Here's how the part is built. I have some questions about the finished solid (model axes, mm). A direction names the side the tool comes from. Round coordinates to 2 decimals unless told otherwise and drop trailing zeros. Write each loop counter-clockwise with the first axis right and the second up, starting at its lowest first coordinate (ties: lowest second). Pieces come first, ordered by that corner, then holes. Notation, with made-up numbers: M 79,-23 L 109,-23 A24 ccw 109,7 Z; hole C 0.5,79.25 d6. An arc over 180 degrees is marked long. Use one line per item in the form item = value. Start each with the question number.
Q1. I'm going to push flat-ended pins straight in: pin 1 Ø1 at (x, z) = (-1.5, 0) entering from -Y; pin 2 Ø1.1 at (x, y) = (-1.5, 7) entering from -Z; pin 3 Ø2 at (x, z) = (2, -0.5) entering from +Y; pin 4 Ø0.7 at (y, z) = (6.5, 1) entering from +X. Where does each tip first touch, or does it pass through?
Q2. I want a section at B-B on z = 0. List the corners of the cut face in (x, y) for me, and give its area (3 significant figures).
Q3. I need wall thicknesses on line 1 along Z through (x, y) = (-0.8, 6.25); line 2 along X through (y, z) = (6.25, -1.1); line 3 along X through (y, z) = (6.5, -1.2). Which ranges of each line are inside material? Lowest first, please. Write a range as from..to.
Q4. I want a section at D-D on z = -0.75. List the corners of the cut face in (x, y) for me.
Q5. We'd pull the mould along X, two halves only. Please class faces 5 (the face through (1, 7, -0.5)), 6 (the face through (0.5, 7, -1)), 7 (the face through (-1.5, 2.46, -0.07)): +X half, -X half, draft (parallel to the pull), parting line (faces both ways), or undercut.
Q6. For faces 1 (the face through (0, 0, 0)), 2 (the face through (0.5, 7, 1)), 3 (the face through (1, 7, 0.5)), 4 (the face through (2, 5, 0)), which set-ups out of +Z, -Z, +X, -X, +Y, -Y let a thin tool reach every point of the face, with its end or its side?
Q7. I want a section at A-A on x = 0. List the corners of the cut face in (y, z) for me.
Q8. I want a section at C-C on y = 2.75. List the corners of the cut face in (x, z) for me.
```python
from build123d import *

# Parameters (mm, degrees)
SKETCH1_R           = 1.5
BOSS_EXTRUDE1_DEPTH = 5
REVOLVE1_ANGLE      = 180
CUT_EXTRUDE1_DEPTH  = 2


with BuildPart() as part:
    # Sketch1 → Boss-Extrude1 (new body)
    with BuildSketch(Plane(origin=(0, 0, 0), x_dir=(1, 0, 0), z_dir=(0, 1, 0))):
        Circle(SKETCH1_R)
    extrude(amount=BOSS_EXTRUDE1_DEPTH)

    # Sketch2 → Revolve1 (revolve)
    with BuildSketch(Plane(origin=(0, 5, 0), x_dir=(1, 0, 0), z_dir=(0, 1, 0))):
        with BuildLine():
            Line((0, 2.5), (0, -2.5))
            ThreePointArc((0, -2.5), (2.5, 0), (0, 2.5))
        make_face()
    revolve(axis=Axis((0, 5, -2.5), (0, 0, 1)), revolution_arc=REVOLVE1_ANGLE)

    # Sketch3 → Cut-Extrude1 (cut)
    with BuildSketch(Plane(origin=(0, 8, 0), x_dir=(1, 0, 0), z_dir=(0, 1, 0))):
        Polygon((-0.5, -0.5), (-0.5, -3.128554583), (0.5, -3.128554583), (0.5, -0.5), (2.950746735, -0.5), (2.950746735, 0.5), (0.5, 0.5), (0.5, 2.871445417), (-0.5, 2.871445417), (-0.5, 0.5), (-3.049253265, 0.5), (-3.049253265, -0.5), align=None)
    extrude(amount=-CUT_EXTRUDE1_DEPTH, mode=Mode.SUBTRACT)


solid = part.part
```
Reported:
q1.pin_1 = 0
q1.pin_2 = -1.56
q1.pin_3 = 7.24
q1.pin_4 = 2.03
q2.outline = M -2.5,5 L -1.5,5 L -1.5,0 L 1.5,0 L 1.5,5 L 2.5,5 A2.5 ccw 2.29,6 L -2.29,6 A2.5 ccw Z
q2.area = 19.9 mm^2
q3.line_1 = -2.01..-0.5, 0.5..2.01
q3.line_2 = -1.86..-0.5, 0.5..1.86
q3.line_3 = -1.6..-0.5, 0.5..1.6
q4.outline = M -2.38,5 L -1.3,5 L -1.3,0 L 1.3,0 L 1.3,5 L 2.38,5 A2.38 ccw 0.5,7.33 L 0.5,6 L -0.5,6 L -0.5,7.33 A2.38 ccw Z
q5.face_5 = draft
q5.face_6 = undercut
q5.face_7 = parting line
q6.face_1 = +Z, -Z, +X, -X, -Y
q6.face_2 = +Z, -Z, +Y
q6.face_3 = +X, -X, +Y
q6.face_4 = -Y
q7.outline = M 0,-1.5 L 5,-1.5 L 5,-2.5 A2.5 ccw 6,-2.29 L 6,2.29 A2.5 ccw 5,2.5 L 5,1.5 L 0,1.5 Z
q8.outline = C 0,0 d3
